Geometry: final body of the model. Coordinates: model frame, mm. Face numbers are marked on the shaded views. A direction names the side the tool comes from. Round coordinates to 2 decimals unless told otherwise and drop trailing zeros. Order: outer loops, then holes, each group sorted by start corner. A loop starts at its lowest first (then second) coordinate and runs counter-clockwise, first axis right, second up. Notation, with made-up numbers: (18, 12) - (63, 12) arc R37 ccw to (63, 50) - close; hole circle Ø3 at (32.5, 43). An arc over 180 degrees is marked (long way). Put each result on its own line as item: value. Start each with the question number.
(1) Material intervals for L1, parallel to X at y = -12.25, z = -9; L2, parallel to X at y = -15.25, z = 9; L3, parallel to Y at x = 2, z = -8, sorted ascending. Write a range as [from, to].
(2) Pin query (flat end, axial travel): P1, Ø8, axis at y = -1, z = 7, coming from the -X side; P2, Ø5, axis at x = -24.5, y = -11.5, coming from the -Z side; P3, Ø5, axis at x = -33.5, z = 1.5, coming from the +Y side; P4, Ø3.5, axis at x = 40, z = 9, coming from the -Y side. Return the tip coordinate at first contact, or that it passes through.
(3) Access query for the marked faces 4, 5, 6, 7 and 8. Directions: +Z, -Z, +X, -X, +Y, -Y. A direction counts if a zero-diameter tool reaches every point of the face in a straight line with its end or side. Return the directions, or none.
(4) Section A-A (z = 9). Output: boundary loops of the cut face in (x, y).
(5) Section C-C (z = 23). Output: boundary loops of the cut face in (x, y).
(6) Pull-direction query (X, two-part tool) for the marked faces 1, 2 and 3; classes: released by +X, released by -X, zero draft, split by the parting line, or undercut.
(7) Section B-B (x = 40). Output: boundary loops of the cut face in (y, z), and give its area (3 significant figures).
(8) Section D-D (x = -35.5). Output: boundary loops of the cut face in (y, z), and give its area (3 significant figures).
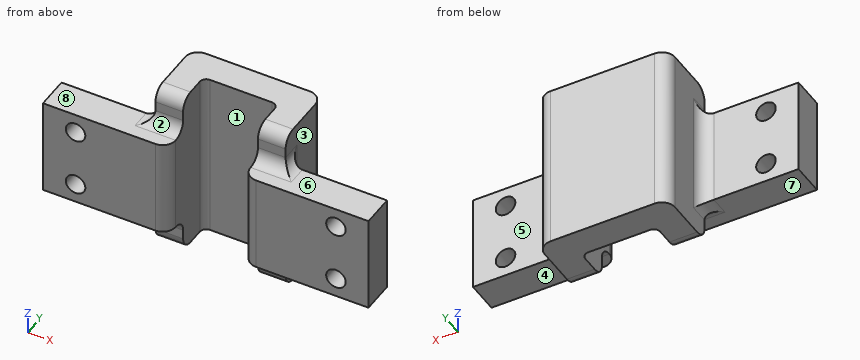
from build123d import *

# Parameters (mm, degrees)
EXTRUDE_1_DEPTH      = 26
EXTRUDE_2_DEPTH      = 8
EXTRUDE_2_DEPTH_BACK = 2
SKETCH_2_W           = 38.5
SKETCH_2_H           = 30
SKETCH_2_R           = 3
FILLET_1_R           = 4
FILLET_2_R           = 4
FILLET_3_R           = 2


with BuildPart() as part:
    # 草圖1 → 填料-伸長1 (new, symmetric)
    with BuildSketch(Plane.XY):
        Polygon((11.5, 1), (11.5, -10), (20, -10), (20, 10), (-20, 10), (-20, -10), (-11.5, -10), (-11.5, 1), align=None)
    extrude(amount=EXTRUDE_1_DEPTH, both=True)

    # 草圖2 → 填料-伸長2 (add, two sides: drawn at the far end of the back side and taken through both)
    # profile 1 of 2: a face of its own
    with BuildSketch(Plane.XZ.offset(10).offset(-EXTRUDE_2_DEPTH_BACK)):
        with Locations((-30.75, 0)):
            Rectangle(SKETCH_2_W, SKETCH_2_H)
        with Locations(Location((-40, 9, 0), (0, 0, 270))):
            Circle(SKETCH_2_R, mode=Mode.SUBTRACT)
        with Locations(Location((-40, -9, 0), (0, 0, 90))):
            Circle(SKETCH_2_R, mode=Mode.SUBTRACT)
    # profile 2 of 2: a face of its own
    with BuildSketch(Plane.XZ.offset(10).offset(-EXTRUDE_2_DEPTH_BACK)):
        with Locations((30.75, 0)):
            Rectangle(SKETCH_2_W, SKETCH_2_H)
        with Locations(Location((40, 9, 0), (0, 0, 90))):
            Circle(SKETCH_2_R, mode=Mode.SUBTRACT)
        with Locations(Location((40, -9, 0), (0, 0, 270))):
            Circle(SKETCH_2_R, mode=Mode.SUBTRACT)
    extrude(amount=EXTRUDE_2_DEPTH + EXTRUDE_2_DEPTH_BACK)

    # 圓角1
    fillet_1_edges = [part.edges().sort_by_distance(p)[0] for p in [
        (20, 10, 0),
        (-20, 10, 0),
        (-11.5, -18, 0),
        (-20, -8, 0),
        (-15.75, -10, -15),
        (15.75, -10, -15),
        (-15.75, -10, 15),
        (15.75, -10, 15),
        (20, -8, 0),
        (11.5, -18, 0),
        (-20, -9, 15),
        (-20, -9, -15),
        (20, -9, -15),
        (20, -9, 15),
    ]]
    fillet(fillet_1_edges, radius=FILLET_1_R - 0.0001)  # a hair under: the kernel refuses the full size

    # 圓角2
    fillet_2_edges = [part.edges().sort_by_distance(p)[0] for p in [
        (-15.75, -10, -26),
        (15.75, -10, 26),
        (15.75, -10, -26),
        (-15.75, -10, 26),
    ]]
    fillet(fillet_2_edges, radius=FILLET_2_R)

    # 圓角3
    fillet_3_edges = [part.edges().sort_by_distance(p)[0] for p in [
        (11.5, 1, 0),
        (-11.5, 1, 0),
    ]]
    fillet(fillet_3_edges, radius=FILLET_3_R)


solid = part.part
Checks:
1. L1: x = [-50, -43], [-37, -11.5], [11.5, 37], [43, 50]
1. L2: x = [-50, -43], [-37, -11.7], [11.7, 37], [43, 50]
1. L3: y = [1, 10]
2. P1: stops at x = -20.13
2. P2: stops at z = -15.54
2. P3: stops at y = -8
2. P4: passes through
3. face 4: -Z, +X, -Y
3. face 5: +Z, -Z, +X, +Y
3. face 6: +Z, +X, -Y
3. face 7: -Z, -X, -Y
3. face 8: +Z, -X, -Y
4. outline: (-50, -18) - (-43, -18) - (-43, -8) - (-50, -8) - close; (-37, -18) - (-15.5, -18) arc R4 ccw to (-11.5, -14) - (-11.5, -1) arc R2 cw to (-9.5, 1) - (9.5, 1) arc R2 cw to (11.5, -1) - (11.5, -14) arc R4 ccw to (15.5, -18) - (37, -18) - (37, -8) - (24, -8) arc R4 cw to (20, -4) - (20, 6) arc R4 ccw to (16, 10) - (-16, 10) arc R4 ccw to (-20, 6) - (-20, -4) arc R4 cw to (-24, -8) - (-37, -8) - close; (43, -18) - (50, -18) - (50, -8) - (43, -8) - close
5. outline: (-20, -9.87) - (-11.5, -9.87) - (-11.5, -1) arc R2 cw to (-9.5, 1) - (9.5, 1) arc R2 cw to (11.5, -1) - (11.5, -9.87) - (20, -9.87) - (20, 6) arc R4 ccw to (16, 10) - (-16, 10) arc R4 ccw to (-20, 6) - close
6. face 1: undercut
6. face 2: zero draft
6. face 3: released by +X
7. outline: (-18, -15) - (-8, -15) - (-8, -12) - (-18, -12) - close; (-18, -6) - (-8, -6) - (-8, 6) - (-18, 6) - close; (-18, 12) - (-8, 12) - (-8, 15) - (-18, 15) - close
7. area: 180 mm²
8. outline: (-18, -15) - (-8, -15) - (-8, 15) - (-18, 15) - close
8. area: 300 mm²
